Verification items for the finished model (mm, model axes). Face numbers are marked on the shaded views. A direction names the side the tool comes from. Give positions to 0.01 mm unless a question says otherwise; leave off trailing zeros. Order: outer loops, then holes, each group sorted by start corner. A loop starts at its lowest first (then second) coordinate and runs counter-clockwise, first axis right, second up. Notation, with made-up numbers: M 4.5,33.5 L 57.5,33.5 A7 ccw 57.5,45.5 Z; hole C 49,2 d7. An arc over 180 degrees is marked long. Answer as a JSON object with one key per item and string values.
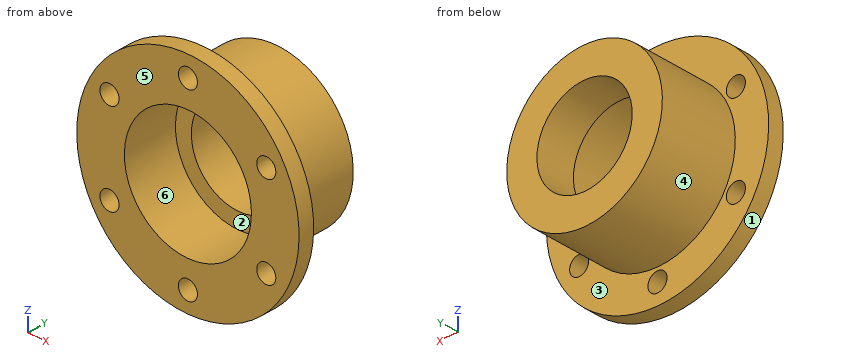
```python
from build123d import *

# Parameters (mm, degrees)
SKETCH2_R          = 3
CUT_EXTRUDE3_DEPTH = 58.879184514


with BuildPart() as part:
    # Sketch1 → Revolve1 (revolve)
    with BuildSketch(Plane.XY, mode=Mode.PRIVATE) as revolve1_sk:
        Polygon((24.5, 0), (35, 0), (35, -5), (20, -5), (20, 12.5), (15, 12.5), (15, 25), (24.5, 25), align=None)
    revolve(revolve1_sk.sketch.rotate(Axis((0, 0, 0), (0, 1, 0)), 90), axis=Axis((0, 0, 0), (0, 1, 0)))

    # Sketch2 → Cut-Extrude3 (cut, through all)
    with BuildSketch(Plane(origin=(0, 25, 0), x_dir=(1, 0, 0), z_dir=(0, 1, 0))):
        with Locations(Location((0, 28.5, 0), (0, 0, 270))):
            Circle(SKETCH2_R)
        with Locations(Location((24.681724008, 14.25, 0), (0, 0, 270))):
            Circle(SKETCH2_R)
        with Locations(Location((24.681724008, -14.25, 0), (0, 0, 270))):
            Circle(SKETCH2_R)
        with Locations(Location((0, -28.5, 0), (0, 0, 270))):
            Circle(SKETCH2_R)
        with Locations(Location((-24.681724008, -14.25, 0), (0, 0, 270))):
            Circle(SKETCH2_R)
        with Locations(Location((-24.681724008, 14.25, 0), (0, 0, 270))):
            Circle(SKETCH2_R)
    extrude(amount=-CUT_EXTRUDE3_DEPTH, mode=Mode.SUBTRACT)


solid = part.part
```
Q1. Gauge pin test, flat ends, axial feed: pin 1 Ø10 at (x, z) = (-18, 24) entering from +Y; pin 2 Ø8 at (x, z) = (0, -28.5) entering from -Y; pin 3 Ø6 at (x, y) = (-8, 16) entering from +Z; pin 4 Ø6 at (x, y) = (-8.5, 12) entering from -Z. Record the tip position at first contact, or that the pin passes through.
Resolved:
{"pin 1": "stops at y = 0", "pin 2": "stops at y = -5", "pin 3": "stops at z = 23.98", "pin 4": "stops at z = -23.87"}
Q2. Section check B-B on z = 3.5. Record the cut outline in (x, y), then the cut area to 3 significant figures.
Resolved:
{"outline": "M -34.82,-5 L -19.69,-5 L -19.69,12.5 L -14.59,12.5 L -14.59,25 L -24.25,25 L -24.25,0 L -34.82,0 Z; M 14.59,12.5 L 19.69,12.5 L 19.69,-5 L 34.82,-5 L 34.82,0 L 24.25,0 L 24.25,25 L 14.59,25 Z", "area": "507 mm²"}
Q3. Section check C-C on x = -23.5. Record the cut outline in (y, z).
Resolved:
{"outline": "M -5,-25.94 L 0,-25.94 L 0,-17.01 L -5,-17.01 Z; M -5,-11.49 L 0,-11.49 L 0,-6.93 L 25,-6.93 L 25,6.93 L 0,6.93 L 0,11.49 L -5,11.49 Z; M -5,17.01 L 0,17.01 L 0,25.94 L -5,25.94 Z"}
Q4. Section check A-A on x = 0. Record the cut outline in (y, z).
Resolved:
{"outline": "M -5,-35 L 0,-35 L 0,-31.5 L -5,-31.5 Z; M -5,-25.5 L 0,-25.5 L 0,-24.5 L 25,-24.5 L 25,-15 L 12.5,-15 L 12.5,-20 L -5,-20 Z; M -5,20 L 12.5,20 L 12.5,15 L 25,15 L 25,24.5 L 0,24.5 L 0,25.5 L -5,25.5 Z; M -5,31.5 L 0,31.5 L 0,35 L -5,35 Z"}
Q5. Material ranges on L1, parallel to X at y = -0.75, z = 16; L2, parallel to Z at x = 0.5, y = 3.75; L3, parallel to X at y = -2, z = -14.25, recorded low to high.
Resolved:
{"L1": "x = -31.13 to -27.12, -22.25 to -12, 12 to 22.25, 27.12 to 31.13", "L2": "z = -24.49 to -19.99, 19.99 to 24.49", "L3": "x = -31.97 to -27.68, -21.68 to -14.03, 14.03 to 21.68, 27.68 to 31.97"}
Q6. Tool access check on the marked faces 1, 2 and 3. Record the directions out of +Z, -Z, +X, -X, +Y, -Y that give a thin tool (end or side, any length) a straight path to the whole face; none if there is none.
Resolved:
{"face 1": "+Y, -Y", "face 2": "-Y", "face 3": "+Y"}
Q7. Section check D-D on y = -1. Record the cut outline in (x, z), then the cut area to 3 significant figures.
Resolved:
{"outline": "C 0,0 d70; hole C -24.68,-14.25 d6; hole C -24.68,14.25 d6; hole C 0,0 d40; hole C 0,-28.5 d6; hole C 0,28.5 d6; hole C 24.68,-14.25 d6; hole C 24.68,14.25 d6", "area": "2,420 mm²"}
Q8. Release check for a two-part mould opening along X. For the marked faces 4, 5 and 6 record: +X half, -X half, draft (parallel to the pull), parting line (faces both ways), or undercut.
Resolved:
{"face 4": "parting line", "face 5": "draft", "face 6": "undercut"}
